Job drawing, mm, ordinate dimensions from the low corner. One solid piece. A direction names the side the tool comes from. Give positions to 0.01 mm unless a question says otherwise; leave off trailing zeros. Order: outer loops, then holes, each group sorted by start corner. A loop starts at its lowest first (then second) coordinate and runs counter-clockwise, first axis right, second up. Notation, with made-up numbers: (61.5, 82.5) - (65.5, 82.5) arc R37 ccw to (65.5, 118.5) - close; hole circle Ø1 at (29, -30.75). An arc over 180 degrees is marked (long way). One line per item, written item: value.
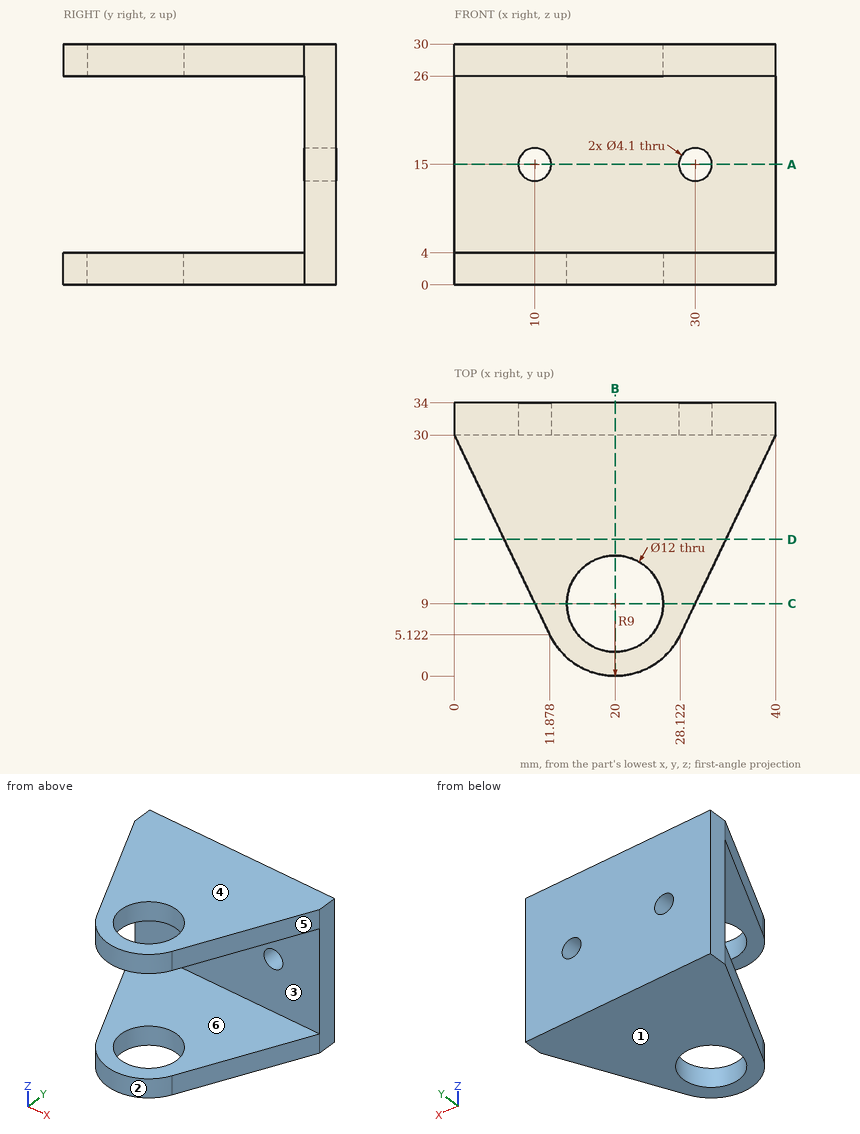
1) Wall check: line 1 along Y through (x, z) = (20, 28.9); line 2 along Z through (x, y) = (8, 26); line 3 along X through (y, z) = (32.8, 15). Give the ranges that are in metal, low to high. Write a range as [from, to].
Answer:
line 1: y = [0, 3], [15, 34]
line 2: z = [0, 4], [26, 30]
line 3: x = [0, 7.95], [12.05, 27.95], [32.05, 40]
2) Which spindle directions (+Z, -Z, +X, -X, +Y, -Y) get a long thin tool onto all of the face, cutting with end or side? Do the marked faces 5 and 6. Say none if no direction does.
Answer:
face 5: +Z, -Z, +X, -Y
face 6: +X, -X, -Y
3) Two-plate mould, pull along Z, no slides. Class the marked faces 1, 2, 3 and 4: pulls with the +Z half, pulls with the -Z half, needs draft (parallel to the pull), parting line crosses it, or undercut.
Answer:
face 1: pulls with the -Z half
face 2: needs draft
face 3: undercut
face 4: pulls with the +Z half
4) Slice it at C-C on y = 9. Write the cut outline in (x, z).
Answer:
outline: (10.03, 0) - (14, 0) - (14, 4) - (10.03, 4) - close; (10.03, 26) - (14, 26) - (14, 30) - (10.03, 30) - close; (26, 0) - (29.97, 0) - (29.97, 4) - (26, 4) - close; (26, 26) - (29.97, 26) - (29.97, 30) - (26, 30) - close
5) Slice it at B-B on x = 20. Write the cut outline in (y, z), then the cut area to 3 significant figures.
Answer:
outline: (0, 0) - (3, 0) - (3, 4) - (0, 4) - close; (0, 26) - (3, 26) - (3, 30) - (0, 30) - close; (15, 0) - (34, 0) - (34, 30) - (15, 30) - (15, 26) - (30, 26) - (30, 4) - (15, 4) - close
area: 264 mm2
6) Drop flat-ended pins along their axis: P1, Ø19, axis at x = 20, y = 9, coming from the +Z side; P2, Ø4, axis at x = 17, z = 14.5, coming from the -Y side. Give the stop position or say it passes through.
Answer:
P1: stops at z = 30
P2: stops at y = 30
7) Slice it at A-A on z = 15. Write the cut outline in (x, y), then the cut area to 3 significant figures.
Answer:
outline: (0, 30) - (7.95, 30) - (7.95, 34) - (0, 34) - close; (12.05, 30) - (27.95, 30) - (27.95, 34) - (12.05, 34) - close; (32.05, 30) - (40, 30) - (40, 34) - (32.05, 34) - close
area: 127 mm2
8) Slice it at D-D on y = 17. Write the cut outline in (x, z), then the cut area to 3 significant figures.
Answer:
outline: (6.21, 0) - (33.79, 0) - (33.79, 4) - (6.21, 4) - close; (6.21, 26) - (33.79, 26) - (33.79, 30) - (6.21, 30) - close
area: 221 mm2
